Autodesk Fusion 360 part; units mm, degrees
sketch "Sketch2" plane through (0, 0, 0) normal (0, 0, 1) x (1, 0, 0)
  line L0 (0, 0) -> (82, 0) construction
  line L1 (0, 0) -> (82, 0) construction
  arc A0 (80.7542, 14.2392) -> (-80.7542, 14.2392) centre (0, 0) ccw
  line L2 (-7.8232, -7.9921) -> (8.1768, -7.9921)
  circle A1 centre (-5.472, 5.4816) radius 1.5
  circle A2 centre (5.528, 5.4816) radius 1.5
  circle A3 centre (-5.472, -5.5184) radius 1.5
  circle A4 centre (5.528, -5.5184) radius 1.5
  line L3 (-75.3224, 17.4571) -> (-7.8232, 5.5552)
  line L4 (2.52, 77.3513) -> (2.52, 8.0079)
  line L5 (-2.5183, 8.0079) -> (-2.5183, 77.3462)
  line L6 (75.3853, 17.8691) -> (8.1768, 6.0184)
  arc A5 (75.3853, 17.8691) -> (2.52, 77.3513) centre (0.0798, -0.0088) ccw
  arc A6 (-2.5183, 77.3462) -> (-75.3224, 17.4571) centre (0.0798, -0.0088) ccw
  line L7 (76.2986, 13.4535) -> (80.7542, 14.2392)
  line L8 (8.1768, 1.4418) -> (76.2986, 13.4535)
  line L9 (-76.1439, 13.4262) -> (-80.7542, 14.2392)
  line L10 (-7.8232, 1.3794) -> (-76.1439, 13.4262)
  line L11 (-7.8232, 8.0079) -> (-7.8232, 5.5552)
  line L12 (-7.8232, 1.3794) -> (-7.8232, -7.9921)
  line L13 (8.1768, 8.0079) -> (2.52, 8.0079)
  line L14 (-2.5183, 8.0079) -> (-7.8232, 8.0079)
  line L15 (8.1768, -7.9921) -> (8.1768, 1.4418)
  line L16 (8.1768, 6.0184) -> (8.1768, 8.0079)
  dimension "d9" = 16
  dimension "d10" = 16
  dimension "d12" = 3
  dimension "d13" = 3
  dimension "d14" = 3
  dimension "d15" = 3
extrude "Extrude1" add sketch "Sketch2" along normal blind 5
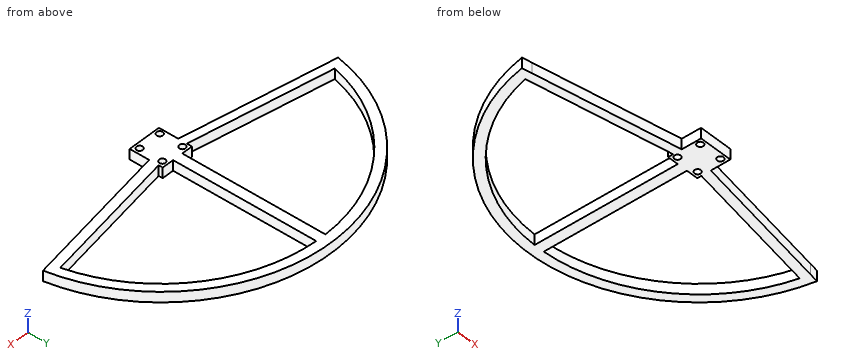
Check sheet for the modelled part. Datum: model origin and axes. Units: mm. Coordinates: 2 decimals unless noted, no trailing zeros. Write each loop counter-clockwise with the first axis right and the second up, starting at its lowest first coordinate (ties: lowest second). Pieces come first, ordered by that corner, then holes. Notation, with made-up numbers: (9.5, 45.5) - (39.5, 45.5) arc R24 cw to (39.5, 84.5) - close; hole circle Ø5 at (12.25, -40). An arc over 180 degrees is marked (long way). One line per question, with ' | ' between items.
Item 1: Sectioned sample at D-D on x = 24.5. Record the boundary of the cut face in (y, z).
Determined:
outline: (4.32, 0) - (8.9, 0) - (8.9, 5) - (4.32, 5) - close; (73.44, 0) - (78.25, 0) - (78.25, 5) - (73.44, 5) - close
Item 2: Thickness scan on line 1 (Y direction, x = -6, z = 0.95); line 2 (X direction, y = 38, z = 4.7); line 3 (X direction, y = 56, z = 4.65). Record the ranges inside material, lowest first. Write a range as [from, to].
Determined:
line 1: y = [-7.99, -6.92], [-4.11, 4.08], [6.89, 8.01], [77.15, 81.78] | line 2: x = [-72.66, -67.34], [-2.52, 2.52], [67.5, 72.66] | line 3: x = [-59.9, -53.34], [-2.52, 2.52], [53.5, 59.9]
Item 3: Sectioned sample at A-A on y = 36.5. Record the boundary of the cut face in (x, z), plus the area to 3 significant figures.
Determined:
outline: (-73.43, 0) - (-68.17, 0) - (-68.17, 5) - (-73.43, 5) - close; (-2.52, 0) - (2.52, 0) - (2.52, 5) - (-2.52, 5) - close; (68.33, 0) - (73.43, 0) - (73.43, 5) - (68.33, 5) - close | area: 77.0 mm2
Item 4: Sectioned sample at C-C on z = 2.9. Record the boundary of the cut face in (x, y).
Determined:
outline: (-80.75, 14.24) - (-76.14, 13.43) - (-7.82, 1.38) - (-7.82, -7.99) - (8.18, -7.99) - (8.18, 1.44) - (76.3, 13.45) - (80.75, 14.24) arc R82 ccw to start; hole (-75.32, 17.46) - (-7.82, 5.56) - (-7.82, 8.01) - (-2.52, 8.01) - (-2.52, 77.35) arc R77.4 ccw to start; hole circle Ø3 at (-5.47, -5.52); hole circle Ø3 at (-5.47, 5.48); hole (2.52, 8.01) - (8.18, 8.01) - (8.18, 6.02) - (75.39, 17.87) arc R77.4 ccw to (2.52, 77.35) - close; hole circle Ø3 at (5.53, -5.52); hole circle Ø3 at (5.53, 5.48)
Item 5: Sectioned sample at B-B on x = -24. Record the boundary of the cut face in (y, z).
Determined:
outline: (4.23, 0) - (8.41, 0) - (8.41, 5) - (4.23, 5) - close; (73.55, 0) - (78.41, 0) - (78.41, 5) - (73.55, 5) - close
Item 6: Gauge pin test, flat ends, axial feed: P1, Ø2, axis at y = 47, z = 3.5, coming from the -X side; P2, Ø2.5, axis at x = 5, z = 2, coming from the +Y side; P3, Ø1.5, axis at y = -4, z = 1.5, coming from the +X side. Record the tip position at first contact, or that the pin passes through.
Determined:
P1: stops at x = -67.88 | P2: stops at y = 81.91 | P3: stops at x = 8.18
